Build history of the part. All positions in model axes, mm. Round coordinates to 2 decimals unless told otherwise and drop trailing zeros. Write each loop counter-clockwise with the first axis right and the second up, starting at its lowest first coordinate (ties: lowest second). Pieces come first, ordered by that corner, then holes. Notation, with made-up numbers: M 30.25,-2.5 L 44.25,-2.5 A11 ccw 44.25,1.5 Z; hole C 41,24.25 d9. An arc over 180 degrees is marked long. Write item = value, one per line. Start each with the question number.
Q1. Band-saw the part on B-B on x = 40. Write the cut outline in (y, z), plus the area to 3 significant figures.
Q2. Drop flat-ended pins along their axis: P1, Ø1.5, axis at y = -2.5, z = 5.5, coming from the -X side; P2, Ø2, axis at x = 33, y = -1.5, coming from the -Z side. Give the stop position or say it passes through.
Q3. Band-saw the part on D-D on x = 2. Write the cut outline in (y, z), plus the area to 3 significant figures.
Q4. Band-saw the part on C-C on y = -1.2. State how many separate pieces and enclosed holes the cut face has, plus the area to 3 significant figures.
Q5. Probe L1, parallel to X at y = -1.8, z = -2; L2, parallel to Z at x = -11, y = -1.65; L3, parallel to X at y = -1.9, z = -9. List the from-to ranges inside material, lowest first.
Q6. Pull direction X, two halves, no side cores. Call faces 1 (the cylindrical face through (7.85, -1.97, -10.35)), 2 (the cylindrical face through (60, -2, 0)), 3 (the flat face through (-28.336, -1.972, -14.628)): released by +X, released by -X, zero draft, split by the parting line, or undercut.
Q7. Band-saw the part on A-A on z = 0. Write the cut outline in (x, y), plus the area to 3 significant figures.
```python
from build123d import *

# Parameters (mm, degrees)
SKETCH_1_R             = 2.1
SKETCH_1_R_2           = 3.1
SM_BASE_FLANGE_1_DEPTH = 4
SKETCH_6_R             = 3.1
CUT_EXTRUDE_1_DEPTH    = 10


# Sheet-metal steps are written as plain solids
with BuildPart() as part:
    # Sketch 1 → Базовая кромка1 (new body)
    with BuildSketch(Plane(origin=(0, 0, 0), x_dir=(1, 0, 0), z_dir=(0, 1, 0))):
        with BuildLine():
            Line((-52, 9.797958971), (-4, 19.595917942))
            ThreePointArc((-4, 19.595917942), (0, 20), (4, 19.595917942))
            Line((4, 19.595917942), (52, 9.797958971))
            ThreePointArc((52, 9.797958971), (60, 0), (52, -9.797958971))
            Line((52, -9.797958971), (4, -19.595917942))
            ThreePointArc((4, -19.595917942), (0, -20), (-4, -19.595917942))
            Line((-4, -19.595917942), (-52, -9.797958971))
            ThreePointArc((-52, -9.797958971), (-60, 0), (-52, 9.797958971))
        make_face()
        with Locations(Location((9.899494937, 9.899494937, 0), (0, 0, 270))):
            Circle(SKETCH_1_R, mode=Mode.SUBTRACT)
        with Locations(Location((9.899494937, -9.899494937, 0), (0, 0, 270))):
            Circle(SKETCH_1_R, mode=Mode.SUBTRACT)
        with Locations(Location((-9.899494937, -9.899494937, 0), (0, 0, 270))):
            Circle(SKETCH_1_R, mode=Mode.SUBTRACT)
        with Locations(Location((-9.899494937, 9.899494937, 0), (0, 0, 270))):
            Circle(SKETCH_1_R, mode=Mode.SUBTRACT)
        with Locations(Location((50, 0, 0), (0, 0, 270))):
            Circle(SKETCH_1_R_2, mode=Mode.SUBTRACT)
        with Locations(Location((-50, 0, 0), (0, 0, 270))):
            Circle(SKETCH_1_R_2, mode=Mode.SUBTRACT)
        with Locations(Location((-40, 0, 0), (0, 0, 270))):
            Circle(SKETCH_1_R_2, mode=Mode.SUBTRACT)
        with Locations(Location((40, 0, 0), (0, 0, 270))):
            Circle(SKETCH_1_R_2, mode=Mode.SUBTRACT)
    extrude(amount=-SM_BASE_FLANGE_1_DEPTH)

    # Эскиз6 → Вырез-Вытянуть1 (cut)
    with BuildSketch(Plane(origin=(0, 0, 0), x_dir=(1, 0, 0), z_dir=(0, 1, 0))):
        with Locations(Location((0, 0, 0), (0, 0, 270))):
            Circle(SKETCH_6_R)
    extrude(amount=-CUT_EXTRUDE_1_DEPTH, mode=Mode.SUBTRACT)


solid = part.part
```
Conclusion:
q1.outline = M -4,-12.25 L 0,-12.25 L 0,-3.1 L -4,-3.1 Z; M -4,3.1 L 0,3.1 L 0,12.25 L -4,12.25 Z
q1.area = 73.2 mm^2
q2.P1 = -58.8
q2.P2 = -13.88
q3.outline = M -4,-19.9 L 0,-19.9 L 0,-2.37 L -4,-2.37 Z; M -4,2.37 L 0,2.37 L 0,19.9 L -4,19.9 Z
q3.area = 140 mm^2
q4.separate_pieces = 1
q4.enclosed_holes = 9
q4.area = 3,170 mm^2
q5.L1 = -59.8 to -52.37, -47.63 to -42.37, -37.63 to -2.37, 2.37 to 37.63, 42.37 to 47.63, 52.37 to 59.8
q5.L2 = -18.17 to -11.69, -8.11 to 8.11, 11.69 to 18.17
q5.L3 = -54.36 to -11.8, -8 to 8, 11.8 to 54.36
q6.face_1 = undercut
q6.face_2 = released by +X
q6.face_3 = released by -X
q7.outline = M -60,-4 L -53.1,-4 L -53.1,0 L -60,0 Z; M -46.9,-4 L -43.1,-4 L -43.1,0 L -46.9,0 Z; M -36.9,-4 L -3.1,-4 L -3.1,0 L -36.9,0 Z; M 3.1,-4 L 36.9,-4 L 36.9,0 L 3.1,0 Z; M 43.1,-4 L 46.9,-4 L 46.9,0 L 43.1,0 Z; M 53.1,-4 L 60,-4 L 60,0 L 53.1,0 Z
q7.area = 356 mm^2
